```python
from build123d import *

# Parameters (mm, degrees)
SKETCH1_R           = 0.5
SKETCH1_R_2         = 0.75
BOSS_EXTRUDE1_DEPTH = 2


with BuildPart() as part:
    # Sketch1 → Boss-Extrude1 (new body)
    with BuildSketch(Plane.XY):
        with BuildLine():
            Line((0, 6), (0, 11.8))
            ThreePointArc((0, 11.8), (1.464466094, 15.335533906), (5, 16.8))
            Line((5, 16.8), (11.2, 16.8))
            ThreePointArc((11.2, 16.8), (14.735533906, 15.335533906), (16.2, 11.8))
            Line((16.2, 11.8), (16.2, 6))
            Line((16.2, 6), (12.2, 6))
            Line((12.2, 6), (12.2, 4))
            Line((12.2, 4), (16.2, 4))
            Line((16.2, 4), (16.2, 2))
            ThreePointArc((16.2, 2), (15.614213562, 0.585786438), (14.2, 0))
            Line((14.2, 0), (2, 0))
            ThreePointArc((2, 0), (0.585786438, 0.585786438), (0, 2))
            Line((0, 2), (0, 4))
            Line((0, 4), (4, 4))
            Line((4, 4), (4, 6))
            Line((4, 6), (0, 6))
        make_face()
        with Locations((3, 13.8)):
            Circle(SKETCH1_R, mode=Mode.SUBTRACT)
        with Locations((13.2, 13.8)):
            Circle(SKETCH1_R, mode=Mode.SUBTRACT)
        with Locations(Location((13.45, 8, 0), (0, 0, 180))):
            Circle(SKETCH1_R_2, mode=Mode.SUBTRACT)
        with Locations(Location((2.75, 8, 0), (0, 0, 180))):
            Circle(SKETCH1_R_2, mode=Mode.SUBTRACT)
        with Locations((13.45, 2)):
            Circle(SKETCH1_R_2, mode=Mode.SUBTRACT)
        with Locations((2.75, 2)):
            Circle(SKETCH1_R_2, mode=Mode.SUBTRACT)
    extrude(amount=BOSS_EXTRUDE1_DEPTH)


solid = part.part
```
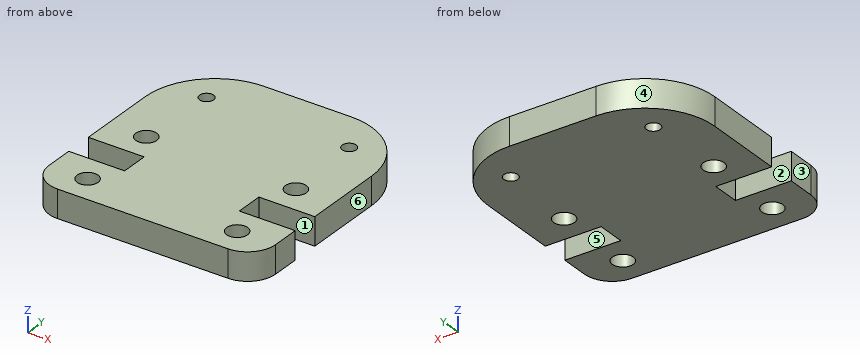
For this review, take the finished solid that the model builds, in its own axes (mm). Face numbers are marked on the shaded views. A direction names the side the tool comes from. Coordinates: 2 decimals unless noted, no trailing zeros. Write each loop counter-clockwise with the first axis right and the second up, starting at its lowest first coordinate (ties: lowest second). Pieces come first, ordered by that corner, then holes. Notation, with made-up numbers: (87, -35) - (115, -35) arc R22 ccw to (115, -11) - close; hole circle Ø4 at (-6, 47.25). An arc over 180 degrees is marked (long way). Put each result on its own line as item: value.
1. Add section D-D, the plane x = 14.5. Give the boundary of the cut face in (y, z), then the cut area to 3 significant figures.
Values found:
outline: (0.02, 0) - (4, 0) - (4, 2) - (0.02, 2) - close; (6, 0) - (15.56, 0) - (15.56, 2) - (6, 2) - close
area: 27.1 mm²
2. Add section A-A, the plane y = 8. Give the boundary of the cut face in (x, z), then the cut area to 3 significant figures.
Values found:
outline: (0, 0) - (2, 0) - (2, 2) - (0, 2) - close; (3.5, 0) - (12.7, 0) - (12.7, 2) - (3.5, 2) - close; (14.2, 0) - (16.2, 0) - (16.2, 2) - (14.2, 2) - close
area: 26.4 mm²
3. Mouldability with a two-part tool opening along Y and no side actions: class the marked faces 4, 5 and 6 as released by +Y, released by -Y, zero draft, split by the parting line, or undercut.
Values found:
face 4: released by +Y
face 5: undercut
face 6: zero draft
4. Machinability: for the marked faces 1, 2 and 3, which of the approach directions +Z, -Z, +X, -X, +Y, -Y give a long, thin tool a straight path to every point of the face, cutting with its end or side? Answer none if there is none.
Values found:
face 1: +Z, -Z, +X
face 2: +Z, -Z, -X
face 3: +Z, -Z, -X, +Y, -Y
5. Wall thickness on probe 1 along X at (y, z) = (8, 0.55); probe 2 along Y at (x, z) = (13.2, 1.15); probe 3 along Y at (x, z) = (2.75, 1.1): over which ranges is each line inside the solid? List them lowest first.
Values found:
probe 1: 0 to 2, 3.5 to 12.7, 14.2 to 16.2
probe 2: 0 to 1.29, 2.71 to 4, 6 to 7.29, 8.71 to 13.3, 14.3 to 16.38
probe 3: 0 to 1.25, 2.75 to 4, 6 to 7.25, 8.75 to 13.37, 14.23 to 16.27
6. Add section B-B, the plane x = 2.75. Give the boundary of the cut face in (y, z).
Values found:
outline: (0, 0) - (1.25, 0) - (1.25, 2) - (0, 2) - close; (2.75, 0) - (4, 0) - (4, 2) - (2.75, 2) - close; (6, 0) - (7.25, 0) - (7.25, 2) - (6, 2) - close; (8.75, 0) - (13.37, 0) - (13.37, 2) - (8.75, 2) - close; (14.23, 0) - (16.27, 0) - (16.27, 2) - (14.23, 2) - close
7. Add section C-C, the plane z = 0.9. Give the boundary of the cut face in (x, y).
Values found:
outline: (0, 2) arc R2 ccw to (2, 0) - (14.2, 0) arc R2 ccw to (16.2, 2) - (16.2, 4) - (12.2, 4) - (12.2, 6) - (16.2, 6) - (16.2, 11.8) arc R5 ccw to (11.2, 16.8) - (5, 16.8) arc R5 ccw to (0, 11.8) - (0, 6) - (4, 6) - (4, 4) - (0, 4) - close; hole circle Ø1.5 at (2.75, 2); hole circle Ø1.5 at (2.75, 8); hole circle Ø1 at (3, 13.8); hole circle Ø1.5 at (13.45, 2); hole circle Ø1.5 at (13.45, 8); hole circle Ø1 at (13.2, 13.8)
8. For pin 1 (0.6 mm diameter, centred on x = 13, z = 1.5, fed in from -Y); pin 2 (1.2 mm diameter, centred on x = 13.45, y = 2, fed in from -Z); pin 3 (0.6 mm diameter, centred on y = 5.5, z = 0.5, fed in from -X); pin 4 (1 mm diameter, centred on x = 2.5, z = 0.5, fed in from +Y), all flat-tipped, find the tip position at first contact; note any pin that passes through.
Values found:
pin 1: y = 0
pin 2: through
pin 3: x = 4
pin 4: y = 16.38
